```python
from build123d import *

# Parameters (mm, degrees)
F0_W      = 100
F0_H      = 200
F1_DEPTH  = 30
F2_R      = 50
F3_DEPTH  = 750
F4_W      = 150
F4_H      = 100
F5_DEPTH  = 650
F6_R      = 50
F7_DEPTH  = 250
F8_W      = 240
F8_H      = 100
F9_DEPTH  = 150
F10_W     = 75
F10_H     = 100
F11_DEPTH = 450
F12_W     = 39.883688
F12_H     = 100
F13_DEPTH = 150
F15_R     = 100
F16_DEPTH = 180


with BuildPart() as f1:
    # F0 (on Top) → F1 (new body)
    with BuildSketch(Plane.XY):
        with Locations((-100, -100)):
            Rectangle(F0_W, F0_H)
    extrude(amount=F1_DEPTH)

    # F2 (on face) → F3 (join)
    with BuildSketch(Plane.XY.offset(30)):
        with Locations((-100, -50)):
            Circle(F2_R)
    extrude(amount=F3_DEPTH)

    # F4 (on face) → F5 (join)
    with BuildSketch(Plane.XY.offset(780)):
        with Locations((-75, -50)):
            Rectangle(F4_W, F4_H)
    extrude(amount=F5_DEPTH)

    # F6 (on face) → F7 (join)
    with BuildSketch(Plane.XY.offset(1430)):
        with Locations((0, -50)):
            Circle(F6_R)
    extrude(amount=F7_DEPTH)

    # F8 (on face) → F9 (join)
    with BuildSketch(Plane.XY.offset(1430)):
        with Locations((-120, -50)):
            Rectangle(F8_W, F8_H)
    extrude(amount=-F9_DEPTH)

    # F10 (on face) → F11 (join)
    with BuildSketch(Plane(origin=(0, 0, 1280), x_dir=(1, 0, 0), z_dir=(0, 0, -1))):
        with Locations((-202.5, 50)):
            Rectangle(F10_W, F10_H)
    extrude(amount=F11_DEPTH)

    # F12 (on face) → F13 (join)
    with BuildSketch(Plane(origin=(0, 0, 830), x_dir=(1, 0, 0), z_dir=(0, 0, -1))):
        with Locations((-199.432023, 50)):
            Rectangle(F12_W, F12_H)
    extrude(amount=F13_DEPTH)

    # F14: F1 across plane


with BuildPart() as f1_1:
    add(f1.part)
    add(f1.part.mirror(Plane.YZ))

    # F15 (on face) → F16 (join)
    with BuildSketch(Plane.XY.offset(1680)):
        with Locations((0, -50)):
            Circle(F15_R)
    extrude(amount=-F16_DEPTH)


solid = f1_1.part
```
Could you check a few things on this model? Use its own coordinates, in mm. A direction names the side the tool comes from. Coordinates: 2 decimals unless noted, no trailing zeros. Loops run counter-clockwise (first coordinate to the right, second up) from the corner with the lowest first, then second, coordinate; pieces in that order, holes last. Notation, with made-up numbers: M 4.25,3.25 L 28.25,3.25 A20 ccw 28.25,11.25 Z; hole C -15.5,60.5 d9. An arc over 180 degrees is marked long. Put each result on its own line as item: value. Start each with the question number.
(1) I need wall thicknesses on line 1 (X direction, y = -45.5, z = 1215); line 2 (Z direction, x = -51, y = -50); line 3 (Z direction, x = -182, y = -11.5). Which ranges of each line are inside material? Lowest first, please. Write a range as from..to.
(2) Suppose I cut it at C-C on x = -202.5. Please give me the cut outline in (y, z).
(3) Suppose I cut it at B-B on z = 561.5. Please give me the cut outline in (x, y).
(4) Will these pins go through, and if not, where does the flat tip stop? P1, Ø4.5, axis at x = -160, y = -31, coming from the -Z side; P2, Ø3, axis at x = 75.5, z = 1179.5, coming from the -Y side; P3, Ø1, axis at x = 60, z = 923.5, coming from the +Y side.
(5) For faces 4 (the face through (179.49, -49, 756)), 5 (the face through (-136.852, -16.208, 399.75)), 6 (the face through (219.374, -49, 756)), 7 (the face through (-140, -88, 780)), 8 (the face through (-140, -12, 30)), which set-ups out of +Z, -Z, +X, -X, +Y, -Y let a thin tool reach every point of the face, with its end or its side?
(6) Suppose I cut it at A-A on z = 935.5. Please give me the cut outline in (x, y), then the cut area to 3 significant figures.
(7) Thinking about a two-plate mould opening in Z: for faces 1 (the face through (101, -141, 30)), 2 (the face through (-50, -101, 15)), 3 (the face through (-101, -99, 0)), which applies, pulls with the +Z half, pulls with the -Z half, needs draft (parallel to the pull), parting line crosses it, or undercut?
Solutions:
1. line 1: x = -240..-165, -150..150, 165..240
1. line 2: z = 0..1430, 1500..1680
1. line 3: z = 680..1430
2. outline: M -100,680 L 0,680 L 0,1430 L -100,1430 Z
3. outline: C -100,-50 d100; C 100,-50 d100
4. P1: stops at z = 1280
4. P2: stops at y = -100
4. P3: stops at y = 0
5. face 4: -Z, +Y, -Y
5. face 5: none
5. face 6: -Z, +X, +Y, -Y
5. face 7: -Y
5. face 8: -X, +Y
6. outline: M -240,-100 L -165,-100 L -165,0 L -240,0 Z; M -150,-100 L 150,-100 L 150,0 L -150,0 Z; M 165,-100 L 240,-100 L 240,0 L 165,0 Z
6. area: 45,000 mm2
7. face 1: undercut
7. face 2: needs draft
7. face 3: pulls with the -Z half
